The model under review builds one solid part; all positions refer to its coordinate system, in mm. Face numbers are marked on the shaded views. A direction names the side the tool comes from. Round coordinates to 2 decimals unless told otherwise and drop trailing zeros. Order: outer loops, then holes, each group sorted by start corner. A loop starts at its lowest first (then second) coordinate and runs counter-clockwise, first axis right, second up. Notation, with made-up numbers: (-30.75, -4.75) - (-18.75, -4.75) arc R10 ccw to (-18.75, 0.25) - close; hole circle Ø8 at (32, 29). An arc over 180 degrees is marked (long way). One line per question, with ' | ' between items. Start each with the question number.
Item 1: Add section A-A on z = 70.5. State the section outline as (x, y) points, and give its area (3 significant figures).
Item 2: For L1, parallel to Y at x = 594, z = 380.5; L2, parallel to X at y = 411, z = 387.5; L3, parallel to Y at x = 549.5, z = 356.5, list the stretches that pass through material, from the lowest coordinate up. Write a range as [from, to].
Item 3: Add section C-C on x = 669.5. State the section outline as (y, z) points.
Item 4: Tool access review of the marked faces 5 and 6: name each direction out of +Z, -Z, +X, -X, +Y, -Y from which nothing blocks a thin tool from reaching the whole face with its end or side.
Item 5: Insertion check: pin 1 Ø12 at (y, z) = (417.5, 162.5) entering from +X; pin 2 Ø8 at (x, z) = (156.5, 198.5) entering from +Y; pin 3 Ø23.5 at (y, z) = (1250.5, 242.5) entering from +X. Each pin has a flat end and moves straight along its axis. Give the tip position at first contact, or say it passes through.
Item 6: Add section B-B on y = 319. State the section outline as (x, z) points.
Item 7: Draft analysis for pull direction Y (two halves, no side actions). For the marked faces 1, 2, 3 and 4, state which applies: +Y half, -Y half, draft (parallel to the pull), parting line (faces both ways), or undercut.
from build123d import *

# Parameters (mm, degrees)
SALIENTE_EXTRUIR3_DEPTH = 500


with BuildPart() as part:
    # Croquis1 → Saliente-Extruir3 (new body)
    with BuildSketch(Plane.XY):
        with BuildLine():
            Line((0, 40.878221652), (0, 0))
            Line((0, 0), (750, 0))
            Line((750, 0), (750, 40.878221652))
            Line((750, 40.878221652), (626.898052252, 40.878221652))
            Line((626.898052252, 40.878221652), (626.898052252, 134.827383306))
            Line((626.898052252, 134.827383306), (576.527963911, 134.827383306))
            Line((576.527963911, 134.827383306), (536.098133641, 175.257213576))
            ThreePointArc((536.098133641, 175.257213576), (525.555715427, 191.210340819), (522.112187733, 210.019566418))
            Line((522.112187733, 210.019566418), (522.112187733, 1186.988416459))
            Line((522.112187733, 1186.988416459), (546.74353007, 1223.418702419))
            Line((546.74353007, 1223.418702419), (626.898052252, 1223.418702419))
            Line((626.898052252, 1223.418702419), (626.898052252, 1301.77405161))
            Line((626.898052252, 1301.77405161), (190.474219634, 1301.77405161))
            Line((190.474219634, 1301.77405161), (190.474219634, 40.878221652))
            Line((190.474219634, 40.878221652), (0, 40.878221652))
        make_face()
    extrude(amount=SALIENTE_EXTRUIR3_DEPTH)


solid = part.part
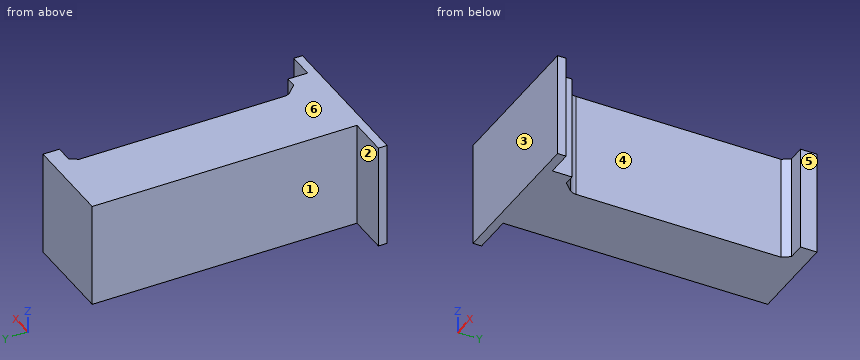
Determined:
1) outline: (0, 0) - (750, 0) - (750, 40.88) - (626.9, 40.88) - (626.9, 134.83) - (576.53, 134.83) - (536.1, 175.26) arc R47.78 cw to (522.11, 210.02) - (522.11, 1186.99) - (546.74, 1223.42) - (626.9, 1223.42) - (626.9, 1301.77) - (190.47, 1301.77) - (190.47, 40.88) - (0, 40.88) - close | area: 469,000 mm2
2) L1: [0, 134.83], [1223.42, 1301.77] | L2: [190.47, 522.11] | L3: [0, 161.86], [1223.42, 1301.77]
3) outline: (0, 0) - (40.88, 0) - (40.88, 500) - (0, 500) - close
4) face 5: +Z, -Z, +X, +Y | face 6: +Z, +X, -X, +Y, -Y
5) pin 1: x = 522.11 | pin 2: y = 40.88 | pin 3: x = 626.9
6) outline: (190.47, 0) - (522.11, 0) - (522.11, 500) - (190.47, 500) - close
7) face 1: draft | face 2: +Y half | face 3: -Y half | face 4: undercut
